Autodesk Inventor part; units mm, degrees
ref_plane "YZ Plane" through (0, 0, 0) normal (1, 0, 0) x (0, 1, 0)
ref_plane "XZ Plane" through (0, 0, 0) normal (0, 1, 0) x (-1, 0, 0)
ref_plane "XY Plane" through (0, 0, 0) normal (0, 0, 1) x (1, 0, 0)
sketch "Sketch1" plane through (0, 0, 0) normal (0, 1, 0) x (-1, 0, 0)
  line L0 (0, 0) -> (55.5, 0)
  line L1 (55.5, 0) -> (55.5, -45)
  line L2 (55.5, -45) -> (0, -45)
  line L3 (0, -45) -> (0, 0)
  dimension "d0" = 55.5
  dimension "d1" = 45
extrude "Extrusion1" add sketch "Sketch1" along normal blind 2
sketch "Sketch2" plane through (0, 0, 0) normal (0, -1, 0) x (1, 0, 0)
  line L0 (0, -45) -> (-55.5, -45)
  line L1 (-55.5, -45) -> (-57, -45)
  line L2 (-57, -45) -> (-57, 0)
  line L3 (-57, 0) -> (-55.5, 0)
  line L4 (-55.5, 0) -> (-55.5, -45)
  line L5 (0, 0) -> (0, -45)
  line L6 (0, -45) -> (1.5, -45)
  line L7 (1.5, -45) -> (1.5, 0)
  line L8 (1.5, 0) -> (0, 0)
  line L9 (0, 0) -> (0, -45)
  dimension "d4" = 1.5
  dimension "d5" = 1.5
extrude "Extrusion2" add sketch "Sketch2" against normal blind 9
sketch "Sketch3" plane through (1.5, 0, 0) normal (1, 0, 0) x (0, 0, -1)
  circle A0 centre (4.5, 4.5) radius 2.15
  line L0 (45, 0) -> (0, 0)
  line L1 (0, 0) -> (0, 9)
  circle A1 centre (40.5, 4.5) radius 2.15
  line L2 (45, 0) -> (45, 9)
  circle A2 centre (22.5, 4.5) radius 2.15
  dimension "d8" = 4.3
  dimension "d9" = 4.5
  dimension "d10" = 4.5
  dimension "d11" = 4.3
  dimension "d12" = 4.5
  dimension "d13" = 4.5
  dimension "d14" = 4.3
hole "Hole1" at (1.5, 4.5, -4.5) at (1.5, 4.5, -22.5) at (1.5, 4.5, -40.5) direction (-1, 0, 0) diameter 4.3 end through all
properties part number "TrolleyBottomPlate"
Build history of the part. All positions in model axes, mm. A direction names the side the tool comes from. Give positions to 0.01 mm unless a question says otherwise; leave off trailing zeros. Loops run counter-clockwise (first coordinate to the right, second up) from the corner with the lowest first, then second, coordinate; pieces in that order, holes last. Notation, with made-up numbers: (67.25, 30) -> (72.25, 30) arc R7 cw to (72.25, 41) -> close; hole circle Ø9 at (1.25, -28.5). An arc over 180 degrees is marked (long way). Answer in a Markdown table with one row per item.
Item 1: Mould opens along Z. For faces 3 (the cylindrical face through (0.74, 5.808, -2.794)), 4 (the flat face through (-28, 1, -45)), 5 (the cylindrical face through (-56.26, 6.41, -23.49)), 6 (the flat face through (0, 7, -22)) say: pulls with the +Z half, pulls with the -Z half, needs draft (parallel to the pull), parting line crosses it, or undercut.
Findings below:
| item | result |
|---|---|
| face 3 | undercut |
| face 4 | pulls with the -Z half |
| face 5 | undercut |
| face 6 | needs draft |
Item 2: Flat gauge pin, fed straight in: P1, Ø2, axis at x = -20.5, z = -36.5, coming from the +Y side. Where does the tip first touch, or does it go through?
Findings below:
| item | result |
|---|---|
| P1 | stops at y = 2 |
Item 3: Probe line 1 along Z through (x, y) = (1.1, 4.5); line 2 along X through (y, z) = (7.25, -3); line 3 along Y through (x, z) = (-56.6, -22.5). List the from-to ranges inside material, lowest first. Write a range as [from, to].
Findings below:
| item | result |
|---|---|
| line 1 | z = [-45, -42.65], [-38.35, -24.65], [-20.35, -6.65], [-2.35, 0] |
| line 2 | x = [-57, -55.5], [0, 1.5] |
| line 3 | y = [0, 2.35], [6.65, 9] |
Item 4: Slice it at C-C on z = -34. Write the cut outline in (x, y).
Findings below:
| item | result |
|---|---|
| outline | (-57, 0) -> (1.5, 0) -> (1.5, 9) -> (0, 9) -> (0, 2) -> (-55.5, 2) -> (-55.5, 9) -> (-57, 9) -> close |
Item 5: Slice it at B-B on y = 4.5. Give the number of separate pieces and of enclosed holes in the cut face, plus the area to 3 significant figures.
Findings below:
| item | result |
|---|---|
| separate pieces | 8 |
| enclosed holes | 0 |
| area | 96.3 mm² |
Item 6: Slice it at A-A on z = -22.5. Write the cut outline in (x, y).
Findings below:
| item | result |
|---|---|
| outline | (-57, 0) -> (1.5, 0) -> (1.5, 2.35) -> (0, 2.35) -> (0, 2) -> (-55.5, 2) -> (-55.5, 2.35) -> (-57, 2.35) -> close; (-57, 6.65) -> (-55.5, 6.65) -> (-55.5, 9) -> (-57, 9) -> close; (0, 6.65) -> (1.5, 6.65) -> (1.5, 9) -> (0, 9) -> close |
Item 7: Tool access for faces 1 (the flat face through (-27, 2, -22)), 2 (the flat face through (1, 9, -22)): list every direction of +Z, -Z, +X, -X, +Y, -Y with a clear straight run to the whole face (end or side of a thin tool).
Findings below:
| item | result |
|---|---|
| face 1 | +Z, -Z, +Y |
| face 2 | +Z, -Z, +X, -X, +Y |
Item 8: Slice it at D-D on y = 7.5. Write the cut outline in (x, z).
Findings below:
| item | result |
|---|---|
| outline | (-57, -45) -> (-55.5, -45) -> (-55.5, 0) -> (-57, 0) -> close; (0, -45) -> (1.5, -45) -> (1.5, 0) -> (0, 0) -> close |
